Geometry: final body of the model. Coordinates: model frame, mm. A direction names the side the tool comes from. Round coordinates to 2 decimals unless told otherwise and drop trailing zeros. Loops run counter-clockwise (first coordinate to the right, second up) from the corner with the lowest first, then second, coordinate; pieces in that order, holes last. Notation, with made-up numbers: (14, 49) - (31, 49) arc R27 ccw to (31, 73) - close; hole circle Ø6 at (-19.75, 0). An arc over 180 degrees is marked (long way). Answer as CSV lines item,"result".
from build123d import *

# Parameters (mm, degrees)
F1_DEPTH = 5
F3_DEPTH = 11
F4_W     = 12.4
F4_H     = 8.4
F5_DEPTH = 20
F6_R     = 2


with BuildPart() as f1:
    # F0 (on Top) → F1 (new body)
    with BuildSketch(Plane.XY):
        with BuildLine():
            Line((0, 42), (0, 0))
            Line((0, 0), (20, 0))
            Line((20, 0), (20, 42))
            ThreePointArc((20, 42), (18.535534, 45.535534), (15, 47))
            ThreePointArc((15, 47), (14.292893, 46.707107), (14, 46))
            Line((14, 46), (14, 39))
            ThreePointArc((14, 39), (10, 35), (6, 39))
            Line((6, 39), (6, 46))
            ThreePointArc((6, 46), (5.707107, 46.707107), (5, 47))
            ThreePointArc((5, 47), (1.464466, 45.535534), (0, 42))
        make_face()
    extrude(amount=F1_DEPTH)

    # F2 (on face) → F3 (join)
    with BuildSketch(Plane.XY.offset(5)):
        with BuildLine():
            Line((0, 24), (0, 0))
            Line((0, 0), (20, 0))
            Line((20, 0), (20, 24))
            ThreePointArc((20, 24), (19.12132, 26.12132), (17, 27))
            Line((17, 27), (3, 27))
            ThreePointArc((3, 27), (0.87868, 26.12132), (0, 24))
        make_face()
    extrude(amount=F3_DEPTH)

    # F4 (on face) → F5 (cut)
    with BuildSketch(Plane.XZ):
        with Locations((10, 8)):
            Rectangle(F4_W, F4_H)
    extrude(amount=-F5_DEPTH, mode=Mode.SUBTRACT)

    # F6
    f6_edges = [f1.edges().sort_by_distance(p)[0] for p in [
        (0, 0, 8),
        (20, 0, 8),
        (20, 12, 16),
        (10, 0, 16),
    ]]
    fillet(f6_edges, radius=F6_R)


solid = f1.part
(1) Section A-A (y = 40). Output: boundary loops of the cut face in (x, z).
Findings below:
outline,"(0, 0) - (6, 0) - (6, 5) - (0, 5) - close; (14, 0) - (20, 0) - (20, 5) - (14, 5) - close"
(2) Access query for faces 1 (the face through (14, 43, 2)), 2 (the face through (10, 27, 9)), 3 (the face through (10, 10, 12.2)), 4 (the face through (0.9, 26.14, 9.44)). Directions: +Z, -Z, +X, -X, +Y, -Y. A direction counts if a zero-diameter tool reaches every point of the face in a straight line with its end or side. Return the directions, or none.
Findings below:
face 1,"+Z, -Z, +Y"
face 2,"+Z, +X, -X, +Y"
face 3,"-Y"
face 4,"+Z, -X, +Y"
(3) Section B-B (z = 13). Output: boundary loops of the cut face in (x, y), and give its area (3 significant figures).
Findings below:
outline,"(0, 2) arc R2 ccw to (2, 0) - (18, 0) arc R2 ccw to (20, 2) - (20, 24) arc R3 ccw to (17, 27) - (3, 27) arc R3 ccw to (0, 24) - close"
area,"534 mm2"
(4) Pin query (flat end, axial travel): P1, Ø7, axis at x = 7, z = 9.5, coming from the +Y side; P2, Ø6, axis at y = 28, z = 10, coming from the -X side; P3, Ø4, axis at y = 35.5, z = 7.5, coming from the -X side; P4, Ø6, axis at x = 5.5, y = 37.5, coming from the +Z side. Return the tip coordinate at first contact, or that it passes through.
Findings below:
P1,"y = 27"
P2,"x = 0.17"
P3,"through"
P4,"z = 5"
(5) Section D-D (y = 8). Output: boundary loops of the cut face in (x, z), and give its area (3 significant figures).
Findings below:
outline,"(0, 0) - (20, 0) - (20, 14) arc R2 ccw to (18, 16) - (2, 16) arc R2 ccw to (0, 14) - close; hole (3.8, 3.8) - (16.2, 3.8) - (16.2, 12.2) - (3.8, 12.2) - close"
area,"214 mm2"
(6) Material intervals for line 1 along X through (y, z) = (17.5, 11.5); line 2 along Z through (x, y) = (6.5, 13.5); line 3 along Y through (x, z) = (15.5, 6.75), sorted ascending.
Findings below:
line 1,"0 to 3.8, 16.2 to 20"
line 2,"0 to 3.8, 12.2 to 16"
line 3,"20 to 27"
(7) Section C-C (x = 10). Output: boundary loops of the cut face in (y, z), and give its area (3 significant figures).
Findings below:
outline,"(0, 0) - (35, 0) - (35, 5) - (27, 5) - (27, 14) arc R2 ccw to (25, 16) - (2, 16) arc R2 ccw to (0, 14) - (0, 12.2) - (20, 12.2) - (20, 3.8) - (0, 3.8) - close"
area,"302 mm2"
(8) Draft query along Z for faces 5 (the face through (10, 20, 8)), 6 (the face through (19.4, 13.15, 15.43)), 7 (the face through (19.14, 26.1, 9.44)). Return one class per face: pulls with the +Z half, pulls with the -Z half, needs draft (parallel to the pull), parting line crosses it, or undercut.
Findings below:
face 5,"undercut"
face 6,"pulls with the +Z half"
face 7,"needs draft"
